Autodesk Inventor part; units mm, degrees
ref_plane "YZ Plane" through (0, 0, 0) normal (1, 0, 0) x (0, 1, 0)
ref_plane "XZ Plane" through (0, 0, 0) normal (0, 1, 0) x (-1, 0, 0)
ref_plane "XY Plane" through (0, 0, 0) normal (0, 0, 1) x (1, 0, 0)
sketch "Sketch1" plane through (0, 0, 0) normal (0, 0, 1) x (1, 0, 0)
  point P0 (0, 0)
sketch "Sketch2" plane through (0, 0, 0) normal (0, 0, 1) x (1, 0, 0)
  line L0 (-25, -25) -> (25, -25)
  line L1 (25, -25) -> (25, 25)
  circle A0 centre (0, 0) radius 12.5
  circle A1 centre (-15.5, 15.5) radius 1.75
  line L2 (25, 25) -> (25, 19)
  line L3 (25, -25) -> (19, -25)
  line L4 (-25, -25) -> (-19, -25)
  circle A2 centre (-15.5, -15.5) radius 1.75
  circle A3 centre (15.5, -15.5) radius 1.75
  circle A4 centre (15.5, 15.5) radius 1.75
  line L5 (-25, 25) -> (-25, 36)
  line L6 (25, 36) -> (25, 25)
  line L7 (0, 36) -> (15, 36)
  line L8 (15, 36) -> (15, 47)
  line L9 (15, 47) -> (21, 47)
  line L10 (21, 47) -> (21, 36)
  line L11 (0, 36) -> (-15, 36)
  line L12 (-15, 36) -> (-15, 47)
  line L13 (-15, 47) -> (-21, 47)
  line L14 (-21, 47) -> (-21, 36)
  circle A5 centre (-36, 0) radius 4
  line L15 (-46, 0) -> (-46, 12.5)
  line L16 (-46, 12.5) -> (-25, 25)
  line L17 (-46, 0) -> (-46, -12.5)
  line L18 (-46, -12.5) -> (-25, -25)
  line L19 (-25, 36) -> (-21, 36)
  line L20 (-15, 36) -> (15, 36)
  line L21 (21, 36) -> (25, 36)
  line L22 (-21, -21) -> (21, -21)
  line L23 (21, -21) -> (21, 21)
  line L24 (21, 21) -> (-21, 21)
  line L25 (-21, 21) -> (-21, -21)
  line L26 (-21, -21) -> (21, 21) construction
  line L27 (21, -21) -> (-21, 21) construction
  dimension "d1" = 50
  dimension "d2" = 25
  dimension "d14" = 3.5
  dimension "d15" = 11
  dimension "d18" = 11
  dimension "d69" = 42
  dimension "d70" = 42
  dimension "d71" = 5.5
  dimension "d72" = 5.5
  dimension "d73" = 5.5
  dimension "d74" = 5.5
  dimension "d75" = 5.5
  dimension "d76" = 5.5
  dimension "d77" = 5.5
  dimension "d78" = 5.5
  dimension "d79" = 8
  dimension "d87" = 36
  dimension "d88" = 46
  dimension "d89" = 25
  dimension "d90" = 50
  dimension "d91" = 50
  dimension "d92" = 15
  dimension "d93" = 6
  dimension "d94" = 4
extrude "Extrusion1" add sketch "Sketch2" against normal blind 25 contours L18 L17 L15 L16 L5 L19 L14 L13 L12 L11 L7 L8 L9 L10 L21 L6 L1 L0 | L25 L24 L23 L22
sketch "Sketch3" plane through (0, 0, 0) normal (0, 1, 0) x (-1, 0, 0)
  point P0 (0, 0)
sketch "Sketch4" plane through (-25, -25, 0) normal (0, -1, 0) x (1, 0, 0)
  point P0 (25, 0)
sketch "Sketch6" plane through (-25, -25, 0) normal (0, -1, 0) x (1, 0, 0)
  line L0 (50, -25) -> (-21, -25)
  line L1 (-21, -25) -> (-21, -12.5)
  line L2 (-21, -12.5) -> (50, -12.5)
  line L3 (50, -12.5) -> (50, -25)
  point P0 (25, 0)
  dimension "d34" = 71
  dimension "d35" = 12.5
extrude "Extrusion2" cut sketch "Sketch6" against normal blind 25
sketch "Sketch7" plane through (25, -25, -12.5) normal (0, 0, -1) x (-1, 0, 0)
  circle A0 centre (40.5, 9.5) radius 1.75
  circle A1 centre (40.5, 9.5) radius 3
  point P0 (25, 25)
  dimension "d38" = 6
extrude "Extrusion3" cut sketch "Sketch7" against normal blind 4 contours A0 | A1
sketch "Sketch8" plane through (25, -25, -12.5) normal (0, 0, -1) x (-1, 0, 0)
  circle A0 centre (9.5, 9.5) radius 1.75
  circle A1 centre (9.5, 9.5) radius 3
  point P0 (25, 25)
  dimension "d44" = 6
extrude "Extrusion4" cut sketch "Sketch8" against normal blind 4 contours A0 | A1
sketch "Sketch9" plane through (0, 0, -25) normal (0, 0, -1) x (-1, 0, 0)
  circle A0 centre (15.5, 15.5) radius 1.75
  circle A1 centre (15.5, 15.5) radius 3
  circle A2 centre (-15.5, 15.5) radius 1.75
  circle A3 centre (-15.5, 15.5) radius 3
  point P0 (0, 0)
  dimension "d47" = 6
  dimension "d48" = 6
extrude "Extrusion5" cut sketch "Sketch9" against normal blind 5 contours A1
sketch "Sketch10" plane through (0, 0, -25) normal (0, 0, -1) x (-1, 0, 0)
  circle A0 centre (-15.5, 15.5) radius 1.75
  circle A1 centre (-15.5, 15.5) radius 3
  point P0 (0, 0)
  dimension "d51" = 6
extrude "Extrusion6" cut sketch "Sketch10" against normal blind 5 contours A0 | A1
move faces "Move1" translate (0, 0, -12.5) faces at (-4.8121, -22.7683, -12.5)
sketch "Sketch11" plane through (-25, -25, 0) normal (0, -1, 0) x (1, 0, 0)
  line L0 (0, -25) -> (50, -25)
  line L1 (50, -25) -> (-21, -25)
  line L2 (-21, -25) -> (-21, -12.5)
  line L3 (-21, -12.5) -> (50, -12.5)
  line L4 (50, -12.5) -> (50, -25)
  point P0 (25, 0)
  dimension "d60" = 71
  dimension "d61" = 12.5
extrude "Extrusion7" cut sketch "Sketch11" against normal blind 15
sketch "Sketch12" plane through (-25, -10, 0) normal (0, -1, 0) x (1, 0, 0)
  line L0 (50, -12.5) -> (50, -25)
  line L1 (50, -25) -> (0, -25)
  line L2 (0, -25) -> (0, -12.5)
  line L3 (0, -12.5) -> (50, -12.5)
  line L4 (50, -12.5) -> (50, -25)
  point P0 (25, 0)
  dimension "d64" = 50
  dimension "d65" = 12.5
extrude "Extrusion8" cut sketch "Sketch12" against normal blind 10
sketch "Sketch13" plane through (-15, 36, 0) normal (0, 1, 0) x (1, 0, 0)
  point P0 (15, 0)
sketch "Sketch14" plane through (-15, 36, 0) normal (0, 1, 0) x (1, 0, 0)
  circle A0 centre (15.5463, 15) radius 3
  point P0 (15, 0)
  dimension "d80" = 6
extrude "Extrusion9" cut sketch "Sketch14" against normal blind 25
ref_plane "Work Plane6" through (-15, 23, 0) normal (0, 1, 0) x (1, 0, 0)
sketch "Sketch15" plane through (-15, 23, 0) normal (0, 1, 0) x (1, 0, 0)
  circle A0 centre (15.5858, 15.0671) radius 5.75
  point P0 (15, 0)
  dimension "d84" = 11.5
extrude "Extrusion10" cut sketch "Sketch15" against normal blind 25
properties part number "SuporteMotor"
Here's how the part is built. I have some questions about the finished solid (model axes, mm). A direction names the side the tool comes from. Coordinates: 2 decimals unless noted, no trailing zeros. Order: outer loops, then holes, each group sorted by start corner. A loop starts at its lowest first (then second) coordinate and runs counter-clockwise, first axis right, second up. Notation, with made-up numbers: M 8.5,-20.75 L 17.5,-20.75 A14 ccw 17.5,3.25 Z; hole C 41.5,38.5 d11. An arc over 180 degrees is marked long. Answer as a JSON object with one key per item and string values. Group by question number.
(1) For pin 1 (1.2 mm diameter, centred on x = -23.5, z = -12.5, fed in from +Y); pin 2 (12 mm diameter, centred on y = 28.5, z = -9, fed in from -X); pin 3 (4 mm diameter, centred on x = -15.5, y = -15.5, fed in from -Z), each with a flat end and sliding along its axis, tell me the tip position at first contact or that it passes through.
(2) Which directions (+Z, -Z, +X, -X, +Y, -Y) give clear straight access to the entire face, cutting with the end or side of a thin tool? Please do faces 4 (the face through (-0.1, 29.59, -12.07)), 5 (the face through (-19, 0, -19)), 6 (the face through (-39.2, -2.4, -12.3)), 7 (the face through (16.15, -12.57, -10.47)), 8 (the face through (5.897, 16.973, -12.865)).
(3) Suppose I cut it at C-C, the plane y = 15.5. Please give me the cut outline in (x, z).
(4) Suppose I cut it at B-B, the plane y = 37.5. Please give me the cut outline in (x, z), then the cut area to 3 significant figures.
(5) I need wall thicknesses on probe 1 along X at (y, z) = (16, -6.75); probe 2 along X at (y, z) = (27.25, -15); probe 3 along X at (y, z) = (-5, -17). Which ranges of each line are inside material? Lowest first, please.
(6) If we mould it in two halves opening along X, with no side actions, what happens to faces 1 (the face through (-13.1, -13.7, -10.5)), 2 (the face through (-46, 0, -12)), 3 (the face through (19, 0, -19))? For each: released by +X, released by -X, zero draft, split by the parting line, or undercut.
(7) Suppose I cut it at D-D, the plane x = -36. Please give me the cut outline in (y, z), then the cut area to 3 significant figures.
(8) Suppose I cut it at A-A, the plane z = -2. Please give me the cut outline in (x, y).
Values found:
{
 "1": {"pin 1": "stops at y = 36", "pin 2": "stops at x = -29.2", "pin 3": "stops at z = -8.5"},
 "2": {"face 4": "+Y", "face 5": "-Z, +X, -Y", "face 6": "+Z, -Z", "face 7": "-Z", "face 8": "none"},
 "3": {"outline": "M -40.96,-25 L -18.5,-25 L -18.5,-20 L -17.25,-20 L -17.25,0 L -40.96,0 Z; M -13.75,-20 L -12.5,-20 L -12.5,-25 L 12.5,-25 L 12.5,-20 L 13.75,-20 L 13.75,0 L -13.75,0 Z; M 17.25,-20 L 18.5,-20 L 18.5,-25 L 25,-25 L 25,0 L 17.25,0 Z; hole C 0.59,-15.07 d11.5"},
 "4": {"outline": "M -21,-25 L -15,-25 L -15,0 L -21,0 Z; M 15,-25 L 21,-25 L 21,0 L 15,0 Z", "area": "300 mm^2"},
 "5": {"probe 1": "x = -40.12 to -17.18, -13.82 to 13.82, 17.18 to 25", "probe 2": "x = -25 to -2.45, 3.55 to 25", "probe 3": "x = -46 to -25"},
 "6": {"face 1": "undercut", "face 2": "released by -X", "face 3": "zero draft"},
 "7": {"outline": "M -18.45,-12.5 L -10,-12.5 L -10,-25 L -4,-25 L -4,0 L -18.45,0 Z; M 4,-25 L 18.45,-25 L 18.45,0 L 4,0 Z", "area": "617 mm^2"},
 "8": {"outline": "M -46,-12.5 L -25,-25 L 25,-25 L 25,36 L 21,36 L 21,47 L 15,47 L 15,36 L -15,36 L -15,47 L -21,47 L -21,36 L -25,36 L -25,25 L -46,12.5 Z; hole C -36,0 d8; hole C -15.5,-15.5 d3.5; hole C -15.5,15.5 d3.5; hole C 0,0 d25; hole C 15.5,-15.5 d3.5; hole C 15.5,15.5 d3.5"}
}
